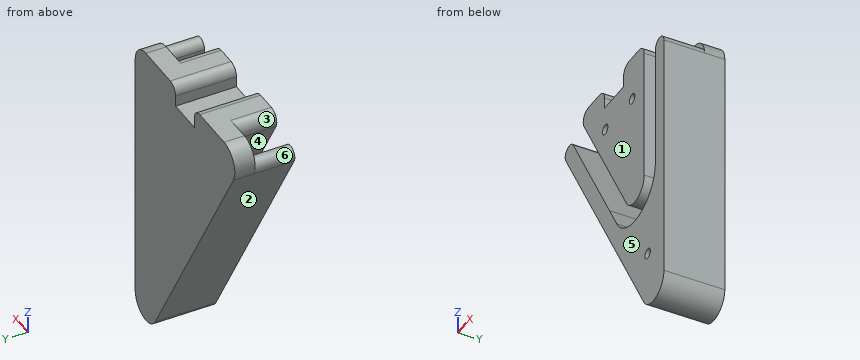
```python
from build123d import *

# Parameters (mm, degrees)
BOSS_EXTRUDE1_DEPTH              = 19.05
SKETCH2_W                        = 11.1125
SKETCH2_H                        = 6.604
CUT_EXTRUDE1_DEPTH               = 112.391012889
CUT_EXTRUDE2_DEPTH               = 12.7
FILLET1_R                        = 3.175
F_1_8_0_125_DIAMETER_HOLE1_D     = 3.175
F_1_8_0_125_DIAMETER_HOLE1_DEPTH = 11.1252
F_1_8_0_125_DIAMETER_HOLE1_TIP   = 0.953866233


with BuildPart() as part:
    # Sketch1 → Boss-Extrude1 (new body)
    with BuildSketch(Plane(origin=(0, 0, 0), x_dir=(1, 0, 0), z_dir=(0, 1, 0))):
        with BuildLine():
            Line((0, 6.35), (0, 86.286703653))
            ThreePointArc((0, 86.286703653), (-4.706499064, 92.420332649), (-11.849261314, 89.461703653))
            Line((-11.849261314, 89.461703653), (-58.000738686, 9.525))
            ThreePointArc((-58.000738686, 9.525), (-58.000738686, 3.175), (-52.501477372, 0))
            Line((-52.501477372, 0), (-6.35, 0))
            ThreePointArc((-6.35, 0), (-1.859871939, 1.859871939), (0, 6.35))
        make_face()
    extrude(amount=BOSS_EXTRUDE1_DEPTH)

    # Sketch2 → Cut-Extrude1 (cut, through all)
    with BuildSketch(Plane(origin=(0, 19.05, 0), x_dir=(1, 0, 0), z_dir=(0, 1, 0))):
        with Locations((-29.425738686, 3.302)):
            Rectangle(SKETCH2_W, SKETCH2_H)
    extrude(amount=-CUT_EXTRUDE1_DEPTH, mode=Mode.SUBTRACT)

    # Sketch3 → Cut-Extrude2 (cut)
    with BuildSketch(Plane(origin=(0, 0, 0), x_dir=(1, 0, 0), z_dir=(0, 1, 0))):
        with BuildLine():
            Line((-22.151280202, 48.250083518), (-50.00847891, 0))
            Line((-50.00847891, 0), (-52.501477372, 0))
            ThreePointArc((-52.501477372, 0), (-58.000738686, 3.175), (-58.000738686, 9.525))
            ThreePointArc((-58.000738686, 9.525), (-57.07103416, 6.055295474), (-53.601329635, 6.985))
            Line((-53.601329635, 6.985), (-32.17376215, 44.098635567))
            Line((-32.17376215, 44.098635567), (-27.870511969, 51.552083518))
            ThreePointArc((-27.870511969, 51.552083518), (-14.132338403, 57.242621331), (-5.08, 45.445384241))
            Line((-5.08, 45.445384241), (-5.08, 36.838883879))
            Line((-5.08, 36.838883879), (-5.08, 6.35))
            ThreePointArc((-5.08, 6.35), (-2.54, 3.81), (0, 6.35))
            ThreePointArc((0, 6.35), (-1.859871939, 1.859871939), (-6.35, 0))
            Line((-6.35, 0), (-11.684, 0))
            Line((-11.684, 0), (-11.684, 45.445384241))
            ThreePointArc((-11.684, 45.445384241), (-15.841579377, 50.863647174), (-22.151280202, 48.250083518))
        make_face()
    extrude(amount=CUT_EXTRUDE2_DEPTH, mode=Mode.SUBTRACT)

    # Fillet1
    fillet1_edges = [part.edges().sort_by_distance(p)[0] for p in [
        (-34.981988686, 9.525, 0),
        (-23.869488686, 9.525, 0),
        (-50.00847891, 6.35, 0),
        (-11.684, 6.35, 0),
    ]]
    fillet(fillet1_edges, radius=FILLET1_R)

    # 1/8 (0.125) Diameter Hole1
    with Locations(Plane(origin=(0, 0, 0), x_dir=(-1, 0, 0), z_dir=(0, -1, 0))):
        with Locations((9.637001873, 74.019445659), (18.796, 14.224), (34.684248681, 14.224)):
            Hole(F_1_8_0_125_DIAMETER_HOLE1_D / 2, depth=F_1_8_0_125_DIAMETER_HOLE1_DEPTH)
            with Locations((0, 0, -(F_1_8_0_125_DIAMETER_HOLE1_DEPTH + F_1_8_0_125_DIAMETER_HOLE1_TIP / 2))):  # 118° drill point
                Cone(0, F_1_8_0_125_DIAMETER_HOLE1_D / 2, F_1_8_0_125_DIAMETER_HOLE1_TIP, mode=Mode.SUBTRACT)


solid = part.part
```
Verification items for the finished model (mm, model axes). Face numbers are marked on the shaded views. A direction names the side the tool comes from. Round coordinates to 2 decimals unless told otherwise and drop trailing zeros. Loops run counter-clockwise (first coordinate to the right, second up) from the corner with the lowest first, then second, coordinate; pieces in that order, holes last. Notation, with made-up numbers: (29, 11) -> (41, 11) arc R27 cw to (41, 50) -> close; hole circle Ø3 at (51, 23.5). An arc over 180 degrees is marked (long way). Answer as a JSON object with one key per item and string values.
Q1. Go/stop test with flat-tipped pins: P1, Ø1, axis at y = 12, z = -5, coming from the +X side; P2, Ø1, axis at x = -17, z = -47, coming from the -Y side; P3, Ø1.9, axis at x = -34.68, z = -14.22, coming from the -Y side; P4, Ø4, axis at y = 7, z = -18, coming from the -X side. Record where each tip stops, or that it passes through.
Data:
{"P1": "stops at x = -0.15", "P2": "stops at y = 0", "P3": "stops at y = 11.5", "P4": "stops at x = -54.26"}
Q2. Section check D-D (x = -41). Record the boundary of the cut face in (y, z), then the cut area to 3 significant figures.
Data:
{"outline": "(0, -38.97) -> (19.05, -38.97) -> (19.05, 0) -> (0, 0) -> (0, -15.6) -> (12.7, -15.6) -> (12.7, -28.81) -> (0, -28.81) -> close", "area": "575 mm2"}
Q3. Section check A-A (y = 16.75). Record the boundary of the cut face in (x, z) (3 decimals).
Data:
{"outline": "(-58.001, -9.525) -> (-11.849, -89.462) arc R6.35 ccw to (0, -86.287) -> (0, -6.35) arc R6.35 ccw to (-6.35, 0) -> (-20.694, 0) arc R3.175 ccw to (-23.869, -3.175) -> (-23.869, -6.604) -> (-34.982, -6.604) -> (-34.982, -3.175) arc R3.175 ccw to (-38.157, 0) -> (-52.501, 0) arc R6.35 ccw to start"}
Q4. Draft check along Z on the marked faces 1, 2, 3 and 4. Enter one of: pulls with the +Z half, pulls with the -Z half, needs draft (parallel to the pull), parting line crosses it, or undercut.
Data:
{"face 1": "needs draft", "face 2": "pulls with the -Z half", "face 3": "undercut", "face 4": "undercut"}
Q5. Section check C-C (z = -56). Record the boundary of the cut face in (x, y).
Data:
{"outline": "(-31.17, 0) -> (-23.44, 0) -> (-23.44, 12.7) -> (-11.15, 12.7) -> (-11.15, 0) -> (0, 0) -> (0, 19.05) -> (-31.17, 19.05) -> close"}
Q6. Access from +Z, -Z, +X, -X, +Y, -Y to the whole of each face (thin tool, end or side, straight path). Record for the marked faces 5 and 6.
Data:
{"face 5": "+Z, -Z, +X, -X, -Y", "face 6": "-Y"}
Q7. Scan lines: line 1 (X direction, y = 10.75, z = -22.5); line 2 (X direction, y = 8.5, z = -44.5); line 3 (X direction, y = 18.25, z = -6). Record each from-to range of solid material in increasing order. Write a range as from..to.
Data:
{"line 1": "x = -50.51..-44.64, -37.02..-11.68, -5.08..0", "line 2": "x = -37.81..-31.94, -24.32..-11.68, -5.08..0", "line 3": "x = -58.84..-34.98, -23.87..-0.01"}
Q8. Section check B-B (y = 4.75). State how many separate pieces and enclosed holes the cut face has, then the cut area to 3 significant figures.
Data:
{"separate pieces": "2", "enclosed holes": "3", "area": "2,390 mm2"}
